Job drawing, mm, ordinate dimensions from the low corner. One solid piece. Give positions to 0.01 mm unless a question says otherwise; leave off trailing zeros. Write each loop counter-clockwise with the first axis right and the second up, starting at its lowest first coordinate (ties: lowest second). Pieces come first, ordered by that corner, then holes. Notation, with made-up numbers: M 88.5,78.25 L 138.5,78.25 A30 cw 138.5,114.25 Z; hole C 42,49 d6. An arc over 180 degrees is marked long. Use CSV: the item, a comma, the result in double quotes. Start each with the question number.
Item 1: Mould opens along Y. For the marked faces 1, 2 and 3 say: released by +Y, released by -Y, zero draft, split by the parting line, or undercut.
Item 2: Cut at D-D (x = 28). List the corners of the cut face in (y, z).
Item 3: Drill centre lines: line 1 (Y direction, x = 51, z = 2); line 2 (X direction, y = 4.25, z = 3.05); line 3 (Y direction, x = 50.5, z = 4.9). Where is each one in solid material? Low to high. Write a range as [from, to].
Item 4: Cut at B-B (x = 51). List the corners of the cut face in (y, z).
Item 5: Cut at A-A (z = 4.95). List the corners of the cut face in (x, y).
Item 6: Cut at C-C (y = 4.5). List the corners of the cut face in (x, z).
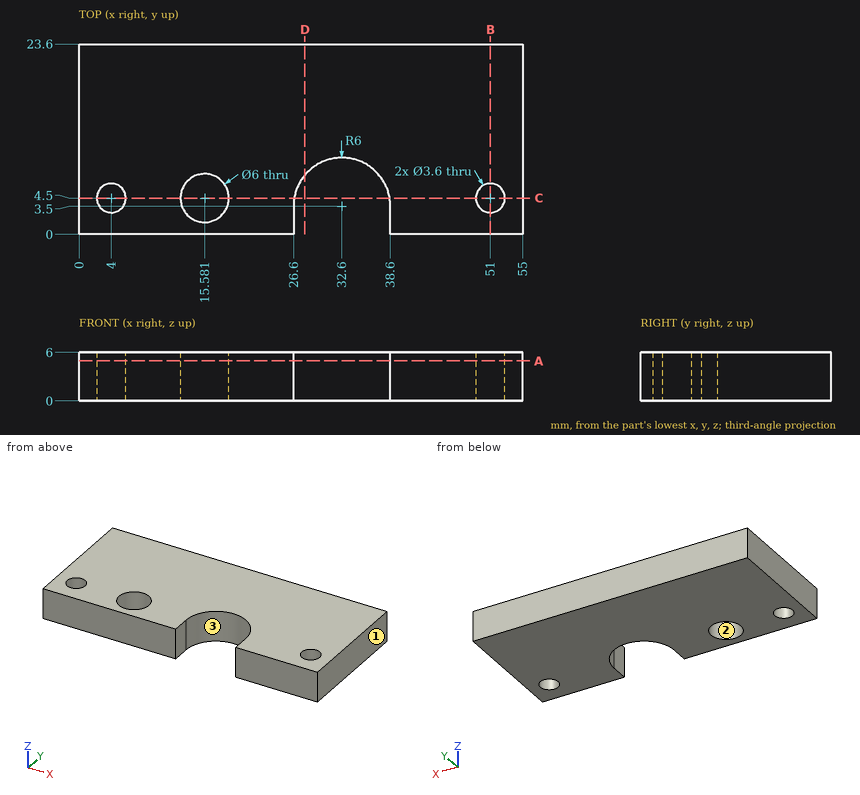
Worked answers:
1,face 1,"zero draft"
1,face 2,"undercut"
1,face 3,"released by -Y"
2,outline,"M 7.35,0 L 23.6,0 L 23.6,6 L 7.35,6 Z"
3,line 1,"y = [0, 2.7], [6.3, 23.6]"
3,line 2,"x = [0, 2.22], [5.78, 12.59], [18.57, 26.65], [38.55, 49.22], [52.78, 55]"
3,line 3,"y = [0, 2.77], [6.23, 23.6]"
4,outline,"M 0,0 L 2.7,0 L 2.7,6 L 0,6 Z; M 6.3,0 L 23.6,0 L 23.6,6 L 6.3,6 Z"
5,outline,"M 0,0 L 26.6,0 L 26.6,3.5 A6 cw 38.6,3.5 L 38.6,0 L 55,0 L 55,23.6 L 0,23.6 Z; hole C 4,4.5 d3.6; hole C 15.58,4.5 d6; hole C 51,4.5 d3.6"
6,outline,"M 0,0 L 2.2,0 L 2.2,6 L 0,6 Z; M 5.8,0 L 12.58,0 L 12.58,6 L 5.8,6 Z; M 18.58,0 L 26.68,0 L 26.68,6 L 18.58,6 Z; M 38.52,0 L 49.2,0 L 49.2,6 L 38.52,6 Z; M 52.8,0 L 55,0 L 55,6 L 52.8,6 Z"
